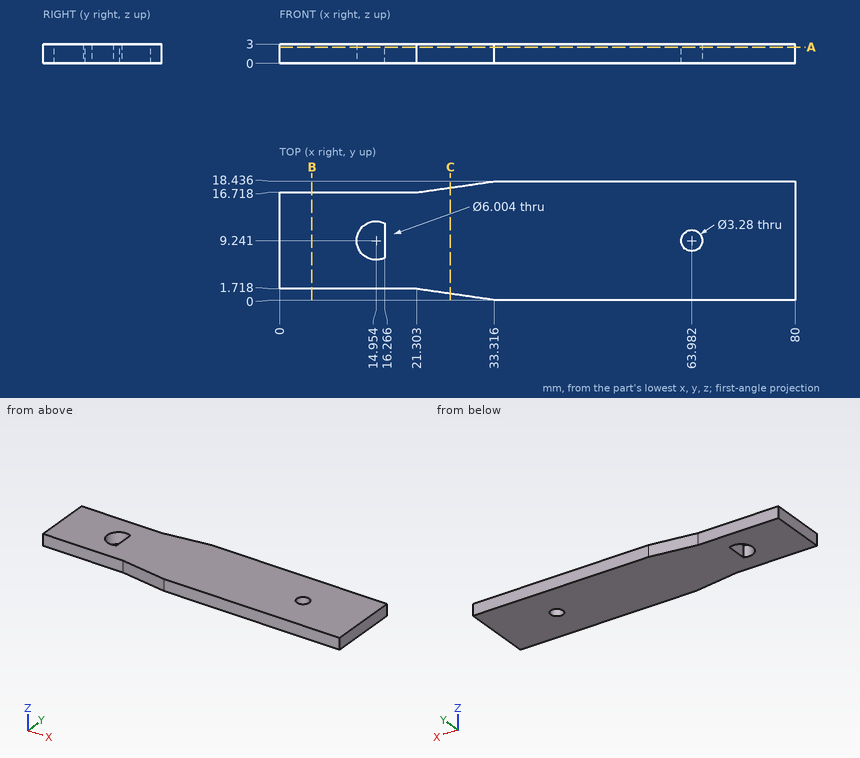
Job drawing, mm, ordinate dimensions from the low corner. One solid piece. Round coordinates to 2 decimals unless told otherwise and drop trailing zeros. Write each loop counter-clockwise with the first axis right and the second up, starting at its lowest first coordinate (ties: lowest second). Pieces come first, ordered by that corner, then holes. Notation, with made-up numbers: (-34, 21.5) -> (-4, 21.5) arc R20 ccw to (-4, 27.5) -> close; hole circle Ø2 at (-16.75, 87). An arc over 180 degrees is marked (long way). Answer as CSV lines item,"result".
1. Slice it at C-C, the plane x = 26.5. List the corners of the cut face in (y, z) (1 decimal).
Resolved:
outline,"(1, 0) -> (17.5, 0) -> (17.5, 3) -> (1, 3) -> close"
2. Slice it at A-A, the plane z = 2.5. List the corners of the cut face in (x, y) (1 decimal), plus the area to 3 significant figures.
Resolved:
outline,"(0, 1.7) -> (21.3, 1.7) -> (33.3, 0) -> (80, 0) -> (80, 18.4) -> (33.3, 18.4) -> (21.3, 16.7) -> (0, 16.7) -> close; hole (16.3, 6.5) -> (16.3, 11.9) arc R3 ccw (long way) to start; hole circle Ø3.3 at (64, 9.2)"
area,"1,350 mm²"
3. Pin check, flat tip, straight feed: pin 1 Ø1.5 at (x, z) = (8, 1.5) entering from -Y. Stop position of the tip, or through.
Resolved:
pin 1,"y = 1.72"
4. Slice it at B-B, the plane x = 5. List the corners of the cut face in (y, z).
Resolved:
outline,"(1.72, 0) -> (16.72, 0) -> (16.72, 3) -> (1.72, 3) -> close"
5. Drill centre lines: line 1 (X direction, y = 9, z = 0.75) (1 decimal); line 2 (Y direction, x = 11, z = 2.35); line 3 (X direction, y = 7.5, z = 1.2) (1 decimal). Where is each one in solid material? Low to high.
Resolved:
line 1,"0 to 12, 16.3 to 62.4, 65.6 to 80"
line 2,"1.72 to 16.72"
line 3,"0 to 12.5, 16.3 to 80"
